from build123d import *

# Parameters (mm, degrees)
SKETCH3_R               = 16.002
BOSS_EXTRUDE1_DEPTH     = 12.7
SKETCH4_R               = 12.7
SKETCH4_R_2             = 10.795
BOSS_EXTRUDE2_DEPTH     = 50.8
CUT_EXTRUDE1_DEPTH      = 56.612660501
CUT_EXTRUDE1_DEPTH_BACK = 56.612660501
SKETCH9_R               = 2.921
CUT_EXTRUDE2_DEPTH      = 68.412002052
CUT_EXTRUDE2_DEPTH_BACK = 68.412002052
SKETCH10_R              = 3.175
CUT_EXTRUDE3_DEPTH      = 4.191
BOSS_EXTRUDE3_DEPTH     = 3.81
SKETCH13_W              = 2.796188768
SKETCH13_H              = 25.396240454
BOSS_EXTRUDE4_DEPTH     = 27.94
SKETCH14_R              = 1
CUT_EXTRUDE4_DEPTH      = 74.166658198
FILLET1_R               = 1.27


with BuildPart() as part:
    # Sketch3 → Boss-Extrude1 (new body)
    with BuildSketch(Plane.XY):
        Circle(SKETCH3_R)
    extrude(amount=BOSS_EXTRUDE1_DEPTH)

    # Sketch4 → Boss-Extrude2 (add)
    with BuildSketch(Plane(origin=(0, 0, 0), x_dir=(-1, 0, 0), z_dir=(0, 0, -1))):
        with Locations(Location((0, 0, 0), (0, 0, 180))):
            Circle(SKETCH4_R)
        Circle(SKETCH4_R_2, mode=Mode.SUBTRACT)
    extrude(amount=BOSS_EXTRUDE2_DEPTH)

    # Sketch9 → Cut-Extrude1 (cut, two sides: drawn at the far end of the back side and taken through both)
    with BuildSketch(Plane(origin=(0, 0, 0), x_dir=(0, 0, -1), z_dir=(1, 0, 0)).offset(-CUT_EXTRUDE1_DEPTH_BACK)):
        with Locations((31.75, 0)):
            Circle(SKETCH9_R)
    extrude(amount=CUT_EXTRUDE1_DEPTH + CUT_EXTRUDE1_DEPTH_BACK, mode=Mode.SUBTRACT)

    # Sketch10 → Cut-Extrude2 (cut, two sides: drawn at the far end of the back side and taken through both)
    with BuildSketch(Plane.XY.offset(12.7).offset(-CUT_EXTRUDE2_DEPTH_BACK)):
        Circle(SKETCH10_R)
    extrude(amount=CUT_EXTRUDE2_DEPTH + CUT_EXTRUDE2_DEPTH_BACK, mode=Mode.SUBTRACT)

    # Sketch5 → Cut-Extrude3 (cut)
    with BuildSketch(Plane(origin=(0, 0, 0), x_dir=(-1, 0, 0), z_dir=(0, 0, -1))):
        Polygon((0, 6.415804866), (-5.55625, 3.207902433), (-5.55625, -3.207902433), (0, -6.415804866), (5.55625, -3.207902433), (5.55625, 3.207902433), align=None)
    extrude(amount=-CUT_EXTRUDE3_DEPTH, mode=Mode.SUBTRACT)

    # Sketch12 → Boss-Extrude3 (add)
    with BuildSketch(Plane.XY.offset(-46.99)):
        with BuildLine():
            Line((36.960470848, -12.7), (36.960470848, 12.7))
            Line((36.960470848, 12.7), (1.105511904, 12.651792104))
            ThreePointArc((1.105511904, 12.651792104), (9.362958965, 8.580501117), (12.7, 0))
            ThreePointArc((12.7, 0), (9.362958965, -8.580501117), (1.105511904, -12.651792104))
            Line((1.105511904, -12.651792104), (36.960470848, -12.7))
        make_face()
    extrude(amount=-BOSS_EXTRUDE3_DEPTH)

    # Sketch13 → Boss-Extrude4 (add)
    with BuildSketch(Plane.XY.offset(-46.99)):
        with Locations((35.562376464, 0.001879773)):
            Rectangle(SKETCH13_W, SKETCH13_H)
    extrude(amount=BOSS_EXTRUDE4_DEPTH)

    # Sketch14 → Cut-Extrude4 (cut, through all)
    with BuildSketch(Plane.ZY.offset(-34.16428208)):
        with Locations((-22.697395511, 10)):
            Circle(SKETCH14_R)
        with Locations(Location((-42.697395511, 10, 0), (0, 0, 180))):
            Circle(SKETCH14_R)
        with Locations((-42.697395511, -10)):
            Circle(SKETCH14_R)
        with Locations(Location((-22.697395511, -10, 0), (0, 0, 180))):
            Circle(SKETCH14_R)
    extrude(amount=-CUT_EXTRUDE4_DEPTH, mode=Mode.SUBTRACT)

    # Fillet1
    fillet1_edges = [part.edges().sort_by_distance(p)[0] for p in [
        (35.562376464, 12.7, -19.05),
        (35.562376464, -12.696240454, -19.05),
    ]]
    fillet(fillet1_edges, radius=FILLET1_R)


solid = part.part
Can you work these out from the model? Positions are in its coordinate system, mm. A direction names the side the tool comes from. Coordinates: 2 decimals unless noted, no trailing zeros. Order: outer loops, then holes, each group sorted by start corner. A loop starts at its lowest first (then second) coordinate and runs counter-clockwise, first axis right, second up. Notation, with made-up numbers: M 82.5,58 L 98.5,58 A21 cw 98.5,79 Z; hole C 2,85.5 d9. An arc over 180 degrees is marked long. Write item = value, one per line.
(1) I need wall thicknesses on line 1 along Z through (x, y) = (11, 0); line 2 along Z through (x, y) = (-4.5, 2.5); line 3 along X through (y, z) = (2.5, -29). Which ranges of each line are inside material? Lowest first, please. Write a range as [from, to].
Results are:
line_1 = [-50.8, -34.67], [-28.83, 12.7]
line_2 = [4.19, 12.7]
line_3 = [-12.45, -10.5], [10.5, 12.45], [34.16, 36.96]
(2) Suppose I cut it at A-A on z = -25.5. Please give me the cut outline in (x, y) (3 decimals).
Results are:
outline = C 0,0 d25.4; M 34.164,-12.696 L 36.96,-12.696 L 36.96,12.7 L 34.164,12.7 Z; hole C 0,0 d21.59
(3) For faces 4 (the face through (35.543, 9.324, -41.96)), 5 (the face through (3, -3, 4.191)), 6 (the face through (11.53, -2.59, -33.1)), 7 (the face through (36, 0, -19.05)), which set-ups out of +Z, -Z, +X, -X, +Y, -Y let a thin tool reach every point of the face, with its end or its side?
Results are:
face_4 = +X
face_5 = -Z
face_6 = -X
face_7 = +Z, +X, +Y, -Y
(4) If we mould it in two halves opening along Y, with no side actions, what happens to faces 1 (the face through (36.96, 0, -35)), 2 (the face through (35.543, -9.956, -43.696)), 3 (the face through (36, -12.696, -34))? For each: pulls with the +Y half, pulls with the -Y half, needs draft (parallel to the pull), parting line crosses it, or undercut.
Results are:
face_1 = needs draft
face_2 = undercut
face_3 = pulls with the -Y half
(5) For pin 1 Ø8 at (x, z) = (-2, -35) entering from -Y; pin 2 Ø10 at (y, z) = (12.5, -41.5) entering from -X; pin 3 Ø12 at (x, y) = (-1, 2) entering from -Z, each with a flat end and sliding along its axis, tell me the tip position at first contact or that it passes through.
Results are:
pin_1 = -12.7
pin_2 = -10.25
pin_3 = 0
(6) Suppose I cut it at D-D on z = -17. Please give me the cut outline in (x, y) (3 decimals), plus the area to 3 significant figures.
Results are:
outline = C 0,0 d25.4; hole C 0,0 d21.59
area = 141 mm2
(7) Suppose I cut it at C-C on y = -10. Please give me the cut outline in (x, z).
Results are:
outline = M -12.49,0 L -7.83,0 L -7.83,-50.8 L -4.07,-50.8 L -4.07,0 L 4.07,0 L 4.07,-50.8 L 36.96,-50.8 L 36.96,-43.7 L 34.16,-43.7 L 34.16,-46.99 L 7.83,-46.99 L 7.83,0 L 12.49,0 L 12.49,12.7 L -12.49,12.7 Z; M 34.16,-41.7 L 36.96,-41.7 L 36.96,-23.7 L 34.16,-23.7 Z; M 34.16,-21.7 L 36.96,-21.7 L 36.96,-19.05 L 34.16,-19.05 Z
(8) Suppose I cut it at B-B on y = 0. State how many separate pieces and enclosed holes the cut face has, plus the area to 3 significant figures.
Results are:
separate_pieces = 4
enclosed_holes = 0
area = 648 mm2
